The model under review builds one solid part; all positions refer to its coordinate system, in mm. A direction names the side the tool comes from. Round coordinates to 2 decimals unless told otherwise and drop trailing zeros. Order: outer loops, then holes, each group sorted by start corner. A loop starts at its lowest first (then second) coordinate and runs counter-clockwise, first axis right, second up. Notation, with made-up numbers: M 14.5,46 L 57.5,46 A15 ccw 57.5,56 Z; hole C -39.75,64 d1. An arc over 180 degrees is marked long. Answer as a JSON object with one key per item and string values. Group by question number.
1. Add section D-D on x = 45.5. State the section outline as (y, z) points, and give its area (3 significant figures).
2. Machinability: for faces 1 (the face through (67.983, -65.175, -9.93)), 2 (the face through (25, -13, -5)), 3 (the face through (0, 33, 0)), 4 (the face through (67.983, -65.175, 10.07)), 5 (the face through (61.63, -49.59, 0.21)), which of the approach directions +Z, -Z, +X, -X, +Y, -Y give a long, thin tool a straight path to every point of the face, cutting with its end or side? Answer none if there is none.
3. Add section B-B on y = 0. State the section outline as (x, z) points.
4. Mouldability with a two-part tool opening along X and no side actions: class faces 6 (the face through (43.389, -64.035, 0.07)), 7 (the face through (3, -10, 15)), 8 (the face through (54.01, -55.69, 0.07)) as released by +X, released by -X, zero draft, split by the parting line, or undercut.
5. Clearance check with flat-ended pins moving along their axes: P1, Ø1, axis at x = 10, z = 1.5, coming from the -Y side; P2, Ø21, axis at x = 37, y = -22.5, coming from the +Z side; P3, Ø3, axis at y = -53.5, z = -0.5, coming from the -X side. State where each tip first meets the part, or that it passes through.
6. Add section C-C on y = -68. State the section outline as (x, z) points, and give its area (3 significant figures).
7. To check wall thickness, follow probe 1 along Y at (x, z) = (0, 8); probe 2 along Y at (x, z) = (1, 5.75); probe 3 along Y at (x, z) = (4.5, 1.5). State the ranges of each line that lie inside material, in increasing order. Write a range as [from, to].
8. Add section A-A on z = -8.5. State the section outline as (x, y) points.
```python
from build123d import *

# Parameters (mm, degrees)
DODANIE_WYCI_GNI_CIE1_DEPTH = 5
SZKIC1_3_R                  = 15
SZKIC1_3_R_2                = 10
DODANIE_WYCI_GNI_CIE2_DEPTH = 15


with BuildPart() as part:
    # Szkic1 → Dodanie-wyci_gni_cie1 (new, symmetric)
    with BuildSketch(Plane.XY):
        with BuildLine():
            Line((0, 49.610742159), (0, 15))
            ThreePointArc((0, 15), (10.606601718, 10.606601718), (15, 0))
            ThreePointArc((15, 0), (10.606601718, -10.606601718), (0, -15))
            Line((0, -15), (17.201404847, -57.569734598))
            Line((17.201404847, -57.569734598), (70.321075739, -70.682872454))
            Line((70.321075739, -70.682872454), (65.579282521, -59.511367123))
            Line((65.579282521, -59.511367123), (42.119104174, -51.763052014))
            Line((42.119104174, -51.763052014), (15, 64.610742159))
            ThreePointArc((15, 64.610742159), (10.606601718, 54.004140441), (0, 49.610742159))
        make_face()
    extrude(amount=DODANIE_WYCI_GNI_CIE1_DEPTH, both=True)

    # Szkic1_3 → Dodanie-wyci_gni_cie2 (add, symmetric)
    # profile 1 of 3: a face of its own
    with BuildSketch(Plane.XY):
        Circle(SZKIC1_3_R)
        Circle(SZKIC1_3_R_2, mode=Mode.SUBTRACT)
    # profile 2 of 3: a face of its own
    with BuildSketch(Plane.XY):
        with Locations((0, 64.610742159)):
            Circle(SZKIC1_3_R)
        with Locations((0, 64.610742159)):
            Circle(SZKIC1_3_R_2, mode=Mode.SUBTRACT)
    # profile 3 of 3: a face of its own
    with BuildSketch(Plane.XY):
        Polygon((65.579282521, -59.511367123), (57.564045894, -39.385959721), (65.579282521, -36.193774991), (88.178535072, -88.35231955), (81.099328917, -91.419597771), (70.321075739, -70.682872454), align=None)
    extrude(amount=DODANIE_WYCI_GNI_CIE2_DEPTH, both=True)


solid = part.part
```
Recorded:
{
 "1": {"outline": "M -64.56,-5 L -52.88,-5 L -52.88,5 L -64.56,5 Z", "area": "117 mm²"},
 "2": {"face 1": "-Z, -X, -Y", "face 2": "-Z", "face 3": "+Z, -Z, -X", "face 4": "+Z, -X, -Y", "face 5": "+Z, -Z"},
 "3": {"outline": "M -15,-15 L -10,-15 L -10,15 L -15,15 Z; M 10,-15 L 15,-15 L 15,-5 L 30.06,-5 L 30.06,5 L 15,5 L 15,15 L 10,15 Z"},
 "4": {"face 6": "released by -X", "face 7": "zero draft", "face 8": "undercut"},
 "5": {"P1": "stops at y = -40.99", "P2": "stops at z = 5", "P3": "stops at x = 14.95"},
 "6": {"outline": "M 59.45,-5 L 69.18,-5 L 69.18,-15 L 79.36,-15 L 79.36,15 L 69.18,15 L 69.18,5 L 59.45,5 Z", "area": "403 mm²"},
 "7": {"probe 1": "y = [-15, -10], [10, 15], [49.61, 54.61], [74.61, 79.61]", "probe 2": "y = [-14.97, -9.95], [9.95, 14.97], [49.64, 54.66], [74.56, 79.58]", "probe 3": "y = [-26.14, -8.93], [8.93, 55.68], [73.54, 78.92]"},
 "8": {"outline": "C 0,0 d30; C 0,64.61 d30; M 57.56,-39.39 L 65.58,-59.51 L 70.32,-70.68 L 81.1,-91.42 L 88.18,-88.35 L 65.58,-36.19 Z; hole C 0,0 d20; hole C 0,64.61 d20"}
}
